from build123d import *

# Parameters (mm, degrees)
SKETCH_1_R               = 7.95
EXTRUDE_1_DEPTH          = 18
CHAMFER_2_SIZE           = 1
SKETCH_4_R               = 18
EXTRUDE_2_DEPTH          = 3
CHAMFER_1_SIZE           = 1
SKETCH_5_R               = 12.5
EXTRUDE_3_DEPTH          = 20
CUT_EXTRUDE_2_DEPTH      = 35.307433597
CUT_EXTRUDE_2_DEPTH_BACK = 35.307433597
SKETCH_9_R               = 3
CUT_EXTRUDE_START        = 20
SKETCH_10_R              = 7.95
CUT_EXTRUDE_3_DEPTH      = 10


with BuildPart() as part:
    # 草图1 → 凸台-拉伸1 (new body)
    with BuildSketch(Plane(origin=(0, 0, 0), x_dir=(1, 0, 0), z_dir=(0, 1, 0))):
        with Locations(Location((0, 0, 0), (0, 0, 270))):
            Circle(SKETCH_1_R)
    extrude(amount=EXTRUDE_1_DEPTH)

    # 倒角2
    chamfer_2_edges = [part.edges().sort_by_distance(p)[0] for p in [
        (0, 18, -7.95),
    ]]
    chamfer(chamfer_2_edges, length=CHAMFER_2_SIZE)

    # 草图4 → 凸台-拉伸2 (add)
    with BuildSketch(Plane(origin=(0, 0, 0), x_dir=(1, 0, 0), z_dir=(0, 1, 0))):
        with Locations(Location((0, 0, 0), (0, 0, 270))):
            Circle(SKETCH_4_R)
    extrude(amount=-EXTRUDE_2_DEPTH)

    # 倒角1
    chamfer_1_edges = [part.edges().sort_by_distance(p)[0] for p in [
        (0, -3, -18),
    ]]
    chamfer(chamfer_1_edges, length=CHAMFER_1_SIZE)

    # 草图5 → 凸台-拉伸3 (add)
    with BuildSketch(Plane(origin=(0, -3, 0), x_dir=(-1, 0, 0), z_dir=(0, -1, 0))):
        with Locations(Location((0, 0, 0), (0, 0, 90))):
            Circle(SKETCH_5_R)
    extrude(amount=EXTRUDE_3_DEPTH)

    # 草图9 → 切除-拉伸2 (cut, two sides: drawn at the far end of the back side and taken through both)
    with BuildSketch(Plane.XY.offset(-CUT_EXTRUDE_2_DEPTH_BACK)):
        with Locations(Location((0, 9.7, 0), (0, 0, 89.999999999))):
            Circle(SKETCH_9_R)
    extrude(amount=CUT_EXTRUDE_2_DEPTH + CUT_EXTRUDE_2_DEPTH_BACK, mode=Mode.SUBTRACT)

    # 草图10 → 切除-拉伸3 (cut)
    with BuildSketch(Plane(origin=(0, -3, 0), x_dir=(-1, 0, 0), z_dir=(0, -1, 0)).offset(CUT_EXTRUDE_START)):
        with Locations(Location((0, 0, 0), (0, 0, 270))):
            Circle(SKETCH_10_R)
    extrude(amount=-CUT_EXTRUDE_3_DEPTH, mode=Mode.SUBTRACT)


solid = part.part
Build history of the part. All positions in model axes, mm. A direction names the side the tool comes from. Give positions to 0.01 mm unless a question says otherwise; leave off trailing zeros. Write each loop counter-clockwise with the first axis right and the second up, starting at its lowest first coordinate (ties: lowest second). Pieces come first, ordered by that corner, then holes. Notation, with made-up numbers: (-17, -34) - (-3, -34) arc R14 cw to (-3, -15) - close; hole circle Ø1 at (-20, 7). An arc over 180 degrees is marked (long way). Use one line per item in the form item = value. Start each with the question number.
1. Band-saw the part on A-A on x = 0. Write the cut outline in (y, z), plus the area to 3 significant figures.
2. Band-saw the part on D-D on y = 11. Write the cut outline in (x, z).
3. Drop flat-ended pins along their axis: pin 1 Ø20.5 at (x, z) = (0, 0) entering from -Y; pin 2 Ø1.5 at (y, z) = (-3.5, -1) entering from -X; pin 3 Ø5 at (x, z) = (0.5, 2) entering from -Y; pin 4 Ø6 at (y, z) = (0, 13.5) entering from -X. Give the stop position or say it passes through.
4. Band-saw the part on B-B on z = 0. Write the cut outline in (x, y), plus the area to 3 significant figures.
5. Probe line 1 (X direction, y = -15, z = 0); line 2 (Y direction, x = -9.5, z = -3.5); line 3 (X direction, y = 9.7, z = 4.75). List the from-to ranges inside material, lowest first. Write a range as [from, to].
6. Two-plate mould, pull along X, no slides. Class faces 1 (the face through (9, -3, -9)), 2 (the face through (4.837, -18.07, -6.309)), 3 (the face through (-3.045, 8.381, 7.344)): released by +X, released by -X, zero draft, split by the parting line, or undercut.
7. Band-saw the part on C-C on y = -14. Write the cut outline in (x, z).
8. 3-axis set-ups, long thin cutter, end or side, ignore diameter. For faces 4 (the face through (-4, 0, 8)), 5 (the face through (-0.1, 6.7, -0.1)), 6 (the face through (3.755, -12.86, -11.923)): which of +Z, -Z, +X, -X, +Y, -Y reach the whole face in a straight line?
Conclusion:
q1.outline = (-23, -12.5) - (-3, -12.5) - (-3, -17) - (-2, -18) - (0, -18) - (0, -7.95) - (6.7, -7.95) - (6.7, 7.95) - (0, 7.95) - (0, 18) - (-2, 18) - (-3, 17) - (-3, 12.5) - (-23, 12.5) - (-23, 7.95) - (-13, 7.95) - (-13, -7.95) - (-23, -7.95) - close; (12.7, -7.95) - (17, -7.95) - (18, -6.95) - (18, 6.95) - (17, 7.95) - (12.7, 7.95) - close
q1.area = 638 mm²
q2.outline = (-2.7, -7.48) - (-2.7, 7.48) arc R7.95 ccw to start; (2.7, -7.48) arc R7.95 ccw to (2.7, 7.48) - close
q3.pin_1 = -23
q3.pin_2 = -17.22
q3.pin_3 = -13
q3.pin_4 = -14.62
q4.outline = (-18, -2) - (-17, -3) - (-12.5, -3) - (-12.5, -23) - (-7.95, -23) - (-7.95, -13) - (7.95, -13) - (7.95, -23) - (12.5, -23) - (12.5, -3) - (17, -3) - (18, -2) - (18, 0) - (7.95, 0) - (7.95, 17) - (6.95, 18) - (-6.95, 18) - (-7.95, 17) - (-7.95, 0) - (-18, 0) - close; hole circle Ø6 at (0, 9.7)
q4.area = 705 mm²
q5.line_1 = [-12.5, -7.95], [7.95, 12.5]
q5.line_2 = [-23, 0]
q5.line_3 = [-6.37, -3], [3, 6.37]
q6.face_1 = zero draft
q6.face_2 = undercut
q6.face_3 = split by the parting line
q7.outline = circle Ø25 at (0, 0); hole circle Ø15.9 at (0, 0)
q8.face_4 = +Y
q8.face_5 = +Z, -Z
q8.face_6 = -Y
